Design review of the part built by this model. Coordinates are the model's own, in mm. Face numbers are marked on the shaded views. A direction names the side the tool comes from. Coordinates: 2 decimals unless noted, no trailing zeros. Write each loop counter-clockwise with the first axis right and the second up, starting at its lowest first coordinate (ties: lowest second). Pieces come first, ordered by that corner, then holes. Notation, with made-up numbers: M 79.25,-1.75 L 136.25,-1.75 A13 cw 136.25,21.25 Z; hole C 32,-31.75 d1. An arc over 180 degrees is marked long. Return JSON: item names as keys, results as strings. Group by question number.
```python
from build123d import *

# Parameters (mm, degrees)
F1_DEPTH = 6.35
F2_R     = 3.175
F3_DEPTH = 6.35


with BuildPart() as f1:
    # F0 (on Top) → F1 (new body)
    with BuildSketch(Plane.XY):
        with BuildLine():
            Line((0, 12.7), (0, 0))
            Line((0, 0), (50.8, 0))
            Line((50.8, 0), (50.8, 12.7))
            add(Edge.make_bspline(
                [(50.8, 12.7), (48.6625255622, 14.6524333598), (44.3991061989, 18.5467686764), (40.1959131853, 14.6454060899), (38.1, 12.7)],
                knots=[0, 0, 0, 0, 0.5013521438, 1, 1, 1, 1], degree=3))
            add(Edge.make_bspline(
                [(38.1, 12.7), (35.2362812476, 15.1247093608), (29.6729807092, 19.8351533876), (35.3467927178, 23.5818985232), (38.1, 25.4)],
                knots=[0, 0, 0, 0, 0.5147517616, 1, 1, 1, 1], degree=3))
            add(Edge.make_bspline(
                [(38.1, 25.4), (39.9179639958, 23.3656390647), (43.6968492215, 19.1369433918), (48.37331205, 23.2603179807), (50.8, 25.4)],
                knots=[0, 0, 0, 0, 0.4810847346, 1, 1, 1, 1], degree=3))
            Line((50.8, 25.4), (50.8, 38.1))
            Line((50.8, 38.1), (33.02, 38.1))
            Line((33.02, 38.1), (33.02, 45.72))
            ThreePointArc((33.02, 45.72), (25.4, 53.34), (17.78, 45.72))
            Line((17.78, 45.72), (17.78, 38.1))
            Line((17.78, 38.1), (0, 38.1))
            Line((0, 38.1), (0, 25.4))
            add(Edge.make_bspline(
                [(0, 25.4), (1.9184660831, 23.4522608086), (5.857149342, 19.4534787537), (10.3801014579, 23.3839796805), (12.7, 25.4)],
                knots=[0, 0, 0, 0, 0.487083108, 1, 1, 1, 1], degree=3))
            add(Edge.make_bspline(
                [(12.7, 12.7), (15.1297413304, 15.1206540979), (19.8306937088, 19.8040249145), (15.0228529426, 23.577087991), (12.7, 25.4)],
                knots=[0, 0, 0, 0, 0.5168615069, 1, 1, 1, 1], degree=3))
            add(Edge.make_bspline(
                [(0, 12.7), (2.1166666667, 14.5722865894), (6.35, 18.3168597683), (10.5833333333, 14.5722865894), (12.7, 12.7)],
                knots=[0, 0, 0, 0, 0.5, 1, 1, 1, 1], degree=3))
        make_face()
    extrude(amount=F1_DEPTH)

    # F2 (on face) → F3 (cut, through all)
    with BuildSketch(Plane.XY.offset(6.35)):
        with Locations((6.5801870078, 5.1745763049)):
            Circle(F2_R)
    extrude(amount=-F3_DEPTH, mode=Mode.SUBTRACT)


solid = f1.part
```
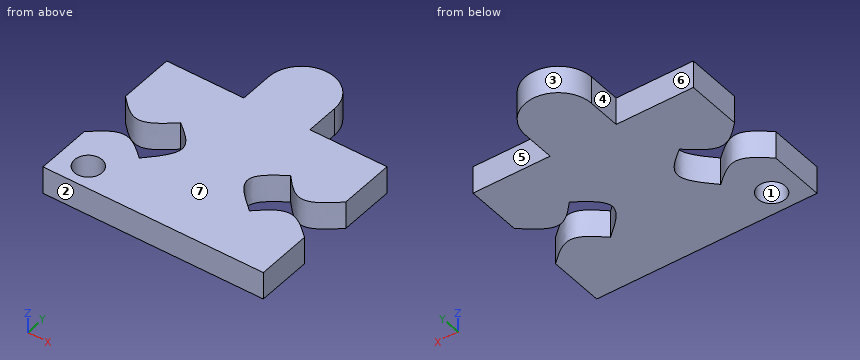
Item 1: Add section B-B (y = 23). Count the separate pieces of the cut face and the enclosed holes in it, plus the area to 3 significant figures.
Item 2: Add section A-A (y = 3). Write out the cut boundary in (x, z), plus the area to 3 significant figures.
Item 3: Add section C-C (x = 22). Write out the cut boundary in (y, z), plus the area to 3 significant figures.
Item 4: For line 1 (X direction, y = 23.5, z = 4.75); line 2 (X direction, y = 43, z = 1.75); line 3 (X direction, y = 6.5, z = 1.25), list the stretches that pass through material, from the lowest coordinate up.
Item 5: The part is to be moulded in two halves that separate along Y. For the marked faces 1, 2, 3 and 4, say which applies: pulls with the +Y half, pulls with the -Y half, needs draft (parallel to the pull), parting line crosses it, or undercut.
Item 6: For pin 1 (1 mm diameter, centred on x = 31.5, z = 3, fed in from +Y); pin 2 (5.5 mm diameter, centred on x = 6.58, y = 5.17, fed in from -Z); pin 3 (3 mm diameter, centred on y = 41.5, z = 4.5, fed in from +X); pin 4 (2 mm diameter, centred on x = 36, z = 4, fed in from +Y), all flat-tipped, find the tip position at first contact; note any pin that passes through.
Item 7: Machinability: for the marked faces 5, 6 and 7, which of the approach directions +Z, -Z, +X, -X, +Y, -Y give a long, thin tool a straight path to every point of the face, cutting with its end or side? Answer none if there is none.
Geometry check:
{
 "1": {"separate pieces": "3", "enclosed holes": "0", "area": "216 mm^2"},
 "2": {"outline": "M 0,0 L 4.27,0 L 4.27,6.35 L 0,6.35 Z; M 8.89,0 L 50.8,0 L 50.8,6.35 L 8.89,6.35 Z", "area": "293 mm^2"},
 "3": {"outline": "M 0,0 L 52.54,0 L 52.54,6.35 L 0,6.35 Z", "area": "334 mm^2"},
 "4": {"line 1": "1.95 to 10.44, 15.02 to 35.35, 39.86 to 48.58", "line 2": "17.78 to 33.02", "line 3": "0 to 3.7, 9.47 to 50.8"},
 "5": {"face 1": "undercut", "face 2": "pulls with the -Y half", "face 3": "pulls with the +Y half", "face 4": "needs draft"},
 "6": {"pin 1": "y = 50.89", "pin 2": "through", "pin 3": "x = 33.02", "pin 4": "y = 38.1"},
 "7": {"face 5": "+Z, -Z, +X, +Y", "face 6": "+Z, -Z, -X, +Y", "face 7": "+Z, +X, -X, +Y, -Y"}
}
